The listing builds one solid part. Answer for the finished solid, in the listing's coordinates (mm). Face numbers are marked on the shaded views. A direction names the side the tool comes from. Coordinates: 2 decimals unless noted, no trailing zeros. Write each loop counter-clockwise with the first axis right and the second up, starting at its lowest first coordinate (ties: lowest second). Pieces come first, ordered by that corner, then holes. Notation, with made-up numbers: M 83,35.5 L 99,35.5 A14 cw 99,55.5 Z; hole C 11.25,-32.75 d6. An arc over 180 degrees is marked long. Answer as CSV lines item,"result".
```python
from build123d import *

# Parameters (mm, degrees)
BOSS_EXTRUDE1_DEPTH = 3
SKETCH2_W           = 24
SKETCH2_H           = 7.62
SKETCH2_R           = 1.551597038
SKETCH2_R_2         = 1.664454239
BOSS_EXTRUDE2_DEPTH = 50.8


with BuildPart() as part:
    # Sketch1 → Boss-Extrude1 (new body)
    with BuildSketch(Plane(origin=(0, 0, 0), x_dir=(1, 0, 0), z_dir=(0, 1, 0))):
        with BuildLine():
            Line((0, 0), (61.5, 0))
            Line((61.5, 0), (61.5, -50.8))
            Line((61.5, -50.8), (0, -50.8))
            Line((0, -50.8), (0, -41.275))
            Line((0, -41.275), (25, -41.275))
            Line((25, -41.275), (25, -38.1))
            ThreePointArc((25, -38.1), (37.7, -25.4), (25, -12.7))
            Line((25, -12.7), (25, -9.525))
            Line((25, -9.525), (0, -9.525))
            Line((0, -9.525), (0, 0))
        make_face()
    extrude(amount=BOSS_EXTRUDE1_DEPTH)

    # Sketch2 → Boss-Extrude2 (add)
    with BuildSketch(Plane(origin=(0, 3, 0), x_dir=(1, 0, 0), z_dir=(0, 1, 0))):
        with Locations((43.75, -46.99)):
            Rectangle(SKETCH2_W, SKETCH2_H)
        with Locations(Location((34.75, -47.245142262, 0), (0, 0, 270))):
            Circle(SKETCH2_R, mode=Mode.SUBTRACT)
        with Locations(Location((52.748191643, -46.99, 0), (0, 0, 270))):
            Circle(SKETCH2_R_2, mode=Mode.SUBTRACT)
    extrude(amount=BOSS_EXTRUDE2_DEPTH)


solid = part.part
```
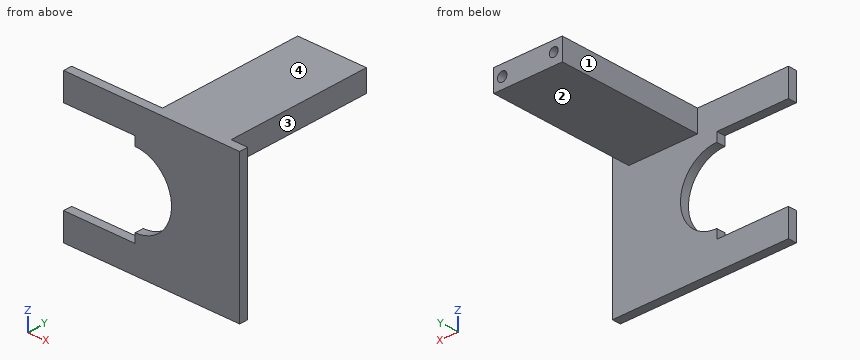
Q1. For the marked faces 1, 2, 3 and 4, determine the directions among +Z, -Z, +X, -X, +Y, -Y from which every point of the face is accessible in a straight line to the end or side of a thin tool.
Output:
face 1,"+Z, -Z, -X, +Y"
face 2,"-Z, +X, -X, +Y"
face 3,"+Z, -Z, +X, +Y"
face 4,"+Z, +X, -X, +Y, -Y"
Q2. Find section D-D (x = 34.75). Give the vertices of the cut face in (y, z), and give its area (3 significant figures).
Output:
outline,"M 0,0 L 3,0 L 3,17.26 L 0,17.26 Z; M 0,33.54 L 3,33.54 L 3,43.18 L 53.8,43.18 L 53.8,45.69 L 3,45.69 L 3,48.8 L 53.8,48.8 L 53.8,50.8 L 0,50.8 Z"
area,"333 mm2"
Q3. Find section C-C (z = 46.99). Give the vertices of the cut face in (x, y), and give its area (3 significant figures).
Output:
outline,"M 0,0 L 61.5,0 L 61.5,3 L 55.75,3 L 55.75,53.8 L 54.41,53.8 L 54.41,3 L 51.08,3 L 51.08,53.8 L 36.28,53.8 L 36.28,3 L 33.22,3 L 33.22,53.8 L 31.75,53.8 L 31.75,3 L 0,3 Z"
area,"1,080 mm2"
Q4. Flat-ended cylindrical pins translate along their axes: pin 1 Ø6 at (y, z) = (18.5, 46.5) entering from -X; pin 2 Ø19 at (x, y) = (39, 23.5) entering from -Z; pin 3 Ø1.5 at (x, z) = (10, 41) entering from +Y. Find the tip coordinate at first contact, or state that the pin passes through.
Output:
pin 1,"x = 31.75"
pin 2,"z = 43.18"
pin 3,"y = 3"
Q5. Find section A-A (x = 6.5). Give the vertices of the cut face in (y, z) (3 decimals).
Output:
outline,"M 0,0 L 3,0 L 3,9.525 L 0,9.525 Z; M 0,41.275 L 3,41.275 L 3,50.8 L 0,50.8 Z"
Q6. Find section B-B (y = 44.5). Give the vertices of the cut face in (x, z), and give its area (3 significant figures).
Output:
outline,"M 31.75,43.18 L 55.75,43.18 L 55.75,50.8 L 31.75,50.8 Z; hole C 34.75,47.25 d3.1; hole C 52.75,46.99 d3.33"
area,"167 mm2"
Q7. Straight lines are drawn through the part: line 1 (X direction, y = 38.5, z = 47); line 2 (X direction, y = 37, z = 46); line 3 (Y direction, x = 21, z = 6). For each, find the intervals that lie inside material, in ascending order.
Output:
line 1,"31.75 to 33.22, 36.28 to 51.08, 54.41 to 55.75"
line 2,"31.75 to 33.82, 35.68 to 51.41, 54.09 to 55.75"
line 3,"0 to 3"
